Verification items for the finished model (mm, model axes). Give positions to 0.01 mm unless a question says otherwise; leave off trailing zeros. Order: outer loops, then holes, each group sorted by start corner. A loop starts at its lowest first (then second) coordinate and runs counter-clockwise, first axis right, second up. Notation, with made-up numbers: (81.25, 55) -> (128.25, 55) arc R5 cw to (128.25, 61) -> close; hole circle Ø8 at (82, 61.5). An arc over 180 degrees is marked (long way). Return JSON: item names as keys, results as strings. Group by question number.
(1) Cross-section at C-C on y = -7. Enter the section's corners in (x, z).
(2) Cross-section at B-B on z = 3.5. State how many separate pieces and enclosed holes the cut face has, then the cut area to 3 significant figures.
(3) Depth check by flat-ended pin: pin 1 Ø4 at (y, z) = (11, 4) entering from +X; pin 2 Ø6 at (x, y) = (-73.5, -14) entering from -Z; pin 3 Ø2.5 at (y, z) = (11, 4) entering from +X; pin 4 Ø4 at (y, z) = (18.5, 5.5) entering from -X. Enter the tip coordinate at first touch or a pass-through.
(4) Thickness scan on line 1 along X through (y, z) = (-24.5, 0.5); line 2 along X through (y, z) = (25, 3.5); line 3 along Y through (x, z) = (-53, 6.25). Record the ranges inside material, lowest first.
(5) Cross-section at A-A on x = 14. Enter the section's corners in (y, z).
from build123d import *

# Parameters (mm, degrees)
F1_DEPTH = 8
F2_R     = 5


with BuildPart() as f1:
    # F0 (on Top) → F1 (new body)
    with BuildSketch(Plane.XY):
        with BuildLine():
            ThreePointArc((-145, -43.026655901), (-141.3409185754, -42.6890851285), (-137.805357045, -41.6877682137))
            Line((-137.805357045, -41.6877682137), (-145, -43.026655901))
        make_face()
        with BuildLine():
            Line((145, -43.026655901), (137.805357045, -41.6877682137))
            ThreePointArc((137.805357045, -41.6877682137), (141.3409185754, -42.6890851285), (145, -43.026655901))
        make_face()
        with BuildLine():
            Line((-137.805357045, -41.6877682137), (-75, -30))
            Line((-75, -30), (-75, 30))
            Line((-75, 30), (-145, -3.026655901))
            ThreePointArc((-145, -3.026655901), (-130.8578643763, -8.8845202772), (-125, -23.026655901))
            ThreePointArc((-125, -23.026655901), (-128.5092016703, -34.3427316541), (-137.805357045, -41.6877682137))
        make_face()
        with BuildLine():
            Line((75, 30), (75, -30))
            Line((75, -30), (137.805357045, -41.6877682137))
            ThreePointArc((137.805357045, -41.6877682137), (125.3375707725, -19.3675744763), (145, -3.026655901))
            Line((145, -3.026655901), (75, 30))
        make_face()
        Polygon((-75, 30), (-75, -30), (-66.3212612271, -30), (75, -30), (75, 30), (43, 30), (43, 0), (35, 0), (35, 30), (-35, 30), (-35, 0), (-43, 0), (-43, 30), align=None)
        with BuildLine():
            Line((-145, -10.526655901), (-145, -3.026655901))
            ThreePointArc((-145, -3.026655901), (-165, -23.026655901), (-145, -43.026655901))
            Line((-145, -43.026655901), (-145, -35.526655901))
            ThreePointArc((-145, -35.526655901), (-151.0104076401, -33.037063541), (-153.5, -27.026655901))
            Line((-153.5, -27.026655901), (-153.5, -19.026655901))
            ThreePointArc((-153.5, -19.026655901), (-151.0104076401, -13.0162482609), (-145, -10.526655901))
        make_face()
        with BuildLine():
            ThreePointArc((165, -23.026655901), (159.1421356237, -8.8845202772), (145, -3.026655901))
            Line((145, -3.026655901), (145, -10.526655901))
            ThreePointArc((145, -10.526655901), (151.0104076401, -13.0162482609), (153.5, -19.026655901))
            Line((153.5, -19.026655901), (153.5, -27.026655901))
            ThreePointArc((153.5, -27.026655901), (151.0104076401, -33.037063541), (145, -35.526655901))
            Line((145, -35.526655901), (145, -43.026655901))
            ThreePointArc((145, -43.026655901), (159.1421356237, -37.1687915247), (165, -23.026655901))
        make_face()
        with BuildLine():
            Line((-145, -43.026655901), (-137.805357045, -41.6877682137))
            ThreePointArc((-137.805357045, -41.6877682137), (-128.5092016703, -34.3427316541), (-125, -23.026655901))
            ThreePointArc((-125, -23.026655901), (-130.8578643763, -8.8845202772), (-145, -3.026655901))
            Line((-145, -3.026655901), (-145, -10.526655901))
            ThreePointArc((-145, -10.526655901), (-138.9895923599, -13.0162482609), (-136.5, -19.026655901))
            Line((-136.5, -19.026655901), (-136.5, -27.026655901))
            ThreePointArc((-136.5, -27.026655901), (-138.9895923599, -33.037063541), (-145, -35.526655901))
            Line((-145, -35.526655901), (-145, -43.026655901))
        make_face()
        with BuildLine():
            ThreePointArc((145, -3.026655901), (125.3375707725, -19.3675744763), (137.805357045, -41.6877682137))
            Line((137.805357045, -41.6877682137), (145, -43.026655901))
            Line((145, -43.026655901), (145, -35.526655901))
            ThreePointArc((145, -35.526655901), (138.9895923599, -33.037063541), (136.5, -27.026655901))
            Line((136.5, -27.026655901), (136.5, -19.026655901))
            ThreePointArc((136.5, -19.026655901), (138.9895923599, -13.0162482609), (145, -10.526655901))
            Line((145, -10.526655901), (145, -3.026655901))
        make_face()
    extrude(amount=F1_DEPTH)

    # F2
    f2_edges = [f1.edges().sort_by_distance(p)[0] for p in [
        (75, -30, 4),
        (-75, -30, 4),
        (-75, 30, 4),
        (75, 30, 4),
        (145, -3.026656, 4),
        (-145, -3.026656, 4),
        (-137.805357, -41.687768, 4),
        (137.805357, -41.687768, 4),
    ]]
    fillet(f2_edges, radius=F2_R)


solid = f1.part
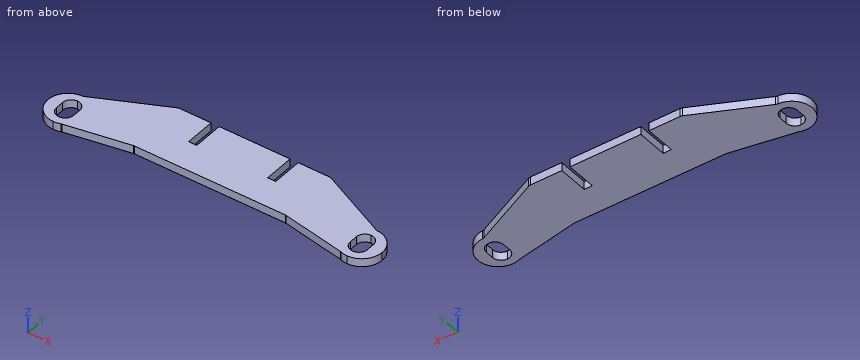
Verdict:
{
 "1": {"outline": "(-156.96, 0) -> (156.96, 0) -> (156.96, 8) -> (-156.96, 8) -> close"},
 "2": {"separate pieces": "1", "enclosed holes": "2", "area": "16,100 mm²"},
 "3": {"pin 1": "x = 119.51", "pin 2": "z = 0", "pin 3": "x = 117.92", "pin 4": "x = -103.61"},
 "4": {"line 1": "-164.95 to -153.5, -136.5 to 136.5, 153.5 to 164.95", "line 2": "-85.6 to -43, -35 to 35, 43 to 85.6", "line 3": "-30 to 30"},
 "5": {"outline": "(-30, 0) -> (30, 0) -> (30, 8) -> (-30, 8) -> close"}
}
